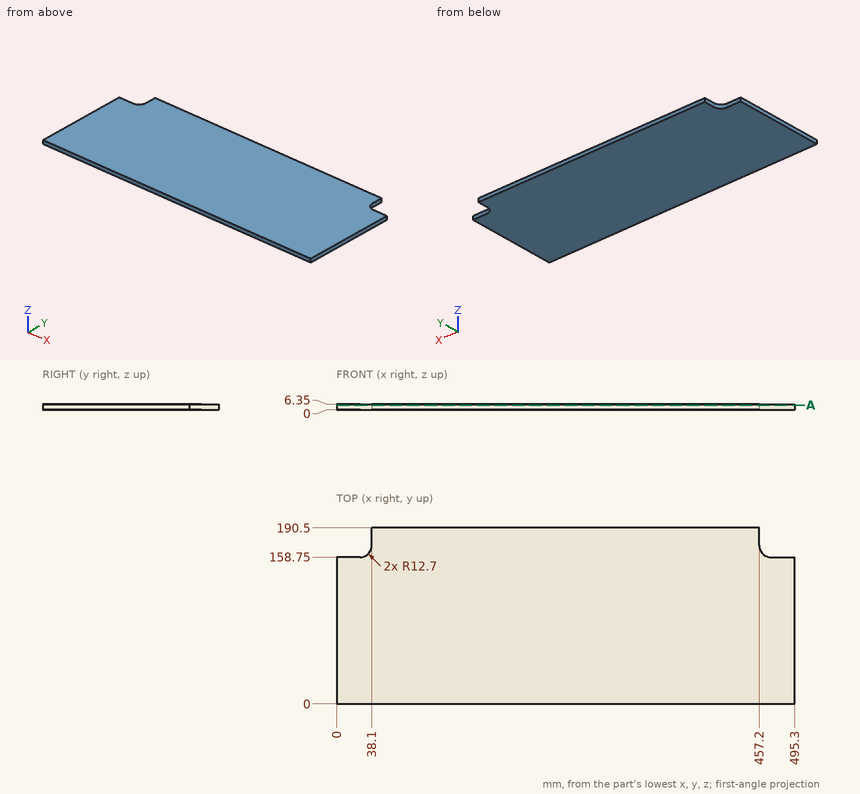
Here's the drawing with two shaded views (mm, measured from the low corner). I have some questions. Round coordinates to 2 decimals unless told otherwise and drop trailing zeros. Order: outer loops, then holes, each group sorted by start corner. A loop starts at its lowest first (then second) coordinate and runs counter-clockwise, first axis right, second up. Notation, with made-up numbers: (35, 26.5) -> (60, 26.5) arc R21 ccw to (60, 59.5) -> close; hole circle Ø5 at (41.5, 12). An arc over 180 degrees is marked (long way). Use a Markdown table: item, result. Add a question column.
(1) For pin 1 Ø3 at (x, z) = (479.5, 2) entering from +Y; pin 2 Ø3 at (y, z) = (184.5, 2.5) entering from -X, each with a flat end and sliding along its axis, tell me the tip position at first contact or that it passes through.
(2) I need wall thicknesses on line 1 along Y through (x, z) = (24.5, 1.25); line 2 along Y through (x, z) = (29.5, 1.5). Which ranges of each line are inside material? Lowest first, please.
(3) Suppose I cut it at A-A, the plane z = 5. Please give me the cut outline in (x, y).
Verdict:
| question | item | result |
|---|---|---|
| 1 | pin 1 | y = 158.75 |
| 1 | pin 2 | x = 38.1 |
| 2 | line 1 | 0 to 158.75 |
| 2 | line 2 | 0 to 159.43 |
| 3 | outline | (0, 0) -> (495.3, 0) -> (495.3, 158.75) -> (469.9, 158.75) arc R12.7 cw to (457.2, 171.45) -> (457.2, 190.5) -> (38.1, 190.5) -> (38.1, 171.45) arc R12.7 cw to (25.4, 158.75) -> (0, 158.75) -> close |
